from build123d import *

# Parameters (mm, degrees)
BOSS_EXTRUDE1_DEPTH            = 6.5
BOSS_EXTRUDE1_DEPTH_BACK       = 3.75
SKETCH1_W                      = 36
SKETCH1_H                      = 48
SKETCH2_W                      = 56
SKETCH2_H                      = 48
BOSS_EXTRUDE2_DEPTH            = 3.75
CBORE_FOR_M3_SHCS1_D           = 3.4
CBORE_FOR_M3_SHCS1_DEPTH       = 10.1
CBORE_FOR_M3_SHCS1_CBORE_D     = 6.5
CBORE_FOR_M3_SHCS1_CBORE_DEPTH = 3
CBORE_FOR_M3_SHCS1_TIP         = 1.021463052
CUT_EXTRUDE1_DEPTH             = 15.25
LPATTERN1_COUNT                = 2
LPATTERN1_PITCH                = 18


with BuildPart() as part:
    # Sketch1 → Boss-Extrude1 (new, two sides: drawn at the far end of the back side and taken through both)
    with BuildSketch(Plane.XY.offset(-BOSS_EXTRUDE1_DEPTH_BACK)):
        Rectangle(SKETCH1_W, SKETCH1_H)
    extrude(amount=BOSS_EXTRUDE1_DEPTH + BOSS_EXTRUDE1_DEPTH_BACK)

    # Sketch2 → Boss-Extrude2 (add)
    with BuildSketch(Plane(origin=(0, 0, 6.5), x_dir=(-1, 0, 0), z_dir=(0, 0, -1))):
        Rectangle(SKETCH2_W, SKETCH2_H)
    extrude(amount=BOSS_EXTRUDE2_DEPTH)

    # CBORE for M3 SHCS1
    with Locations(Plane.XY.offset(6.5)):
        with Locations((-23.5, 17), (-23.5, -17), (23.5, 17), (23.5, -17)):
            CounterBoreHole(CBORE_FOR_M3_SHCS1_D / 2, CBORE_FOR_M3_SHCS1_CBORE_D / 2, CBORE_FOR_M3_SHCS1_CBORE_DEPTH, depth=CBORE_FOR_M3_SHCS1_DEPTH)
            with Locations((0, 0, -(CBORE_FOR_M3_SHCS1_DEPTH + CBORE_FOR_M3_SHCS1_TIP / 2))):  # 118° drill point
                Cone(0, CBORE_FOR_M3_SHCS1_D / 2, CBORE_FOR_M3_SHCS1_TIP, mode=Mode.SUBTRACT)

    # Sketch7 → Cut-Extrude1 (cut)
    with BuildSketch(Plane(origin=(16.5, 0, 0), x_dir=(0, 0, -1), z_dir=(1, 0, 0))):
        Polygon((-6.503383917, 8.006767833), (-3.756779362, 8.006767833), (-3.756779362, 9.003383917), (2.246616083, 9.003383917), (2.246616083, 7.503383917), (3.746616083, 7.503383917), (6.355468839, 7.503383917), (6.355468839, -12.746616083), (3.871124209, -12.746616083), (3.746616083, -12.746616083), (2.246616083, -12.746616083), (2.246616083, -14.496616083), (-3.756779362, -14.496616083), (-3.756779362, -9.25), (-6.503383917, -9.25), align=None)
    cut_extrude1 = extrude(amount=-CUT_EXTRUDE1_DEPTH, mode=Mode.SUBTRACT)

    # LPattern1: Cut-Extrude1 ×2
    with Locations(*[(-i * LPATTERN1_PITCH, 0, 0) for i in range(1, LPATTERN1_COUNT)]):
        add(cut_extrude1, mode=Mode.SUBTRACT)


solid = part.part
Can you work these out from the model? Positions are in its coordinate system, mm. A direction names the side the tool comes from. Round coordinates to 2 decimals unless told otherwise and drop trailing zeros. Order: outer loops, then holes, each group sorted by start corner. A loop starts at its lowest first (then second) coordinate and runs counter-clockwise, first axis right, second up. Notation, with made-up numbers: M 59.5,32.5 L 93.5,32.5 A19 cw 93.5,64.5 Z; hole C -38.75,27.25 d7. An arc over 180 degrees is marked long. Use a Markdown table: item, result.
1) Imagine slicing it at A-A (y = -0.5). List the corners of the cut face in (x, z) for me, then the cut area to 3 significant figures.
Geometry says:
| item | result |
|---|---|
| outline | M -28,2.75 L -18,2.75 L -18,-3.75 L -16.75,-3.75 L -16.75,6.5 L -28,6.5 Z; M -1.5,-3.75 L 1.25,-3.75 L 1.25,6.5 L -1.5,6.5 Z; M 16.5,-3.75 L 18,-3.75 L 18,2.75 L 28,2.75 L 28,6.5 L 16.5,6.5 Z |
| area | 131 mm² |
2) If we mould it in two halves opening along Y, with no side actions, what happens to faces 1 (the face through (-22.1, 15.6, 3.5)), 2 (the face through (28, 0, 5)), 3 (the face through (-9, 9.003, 1))? For each: +Y half, -Y half, draft (parallel to the pull), parting line (faces both ways), or undercut.
Geometry says:
| item | result |
|---|---|
| face 1 | undercut |
| face 2 | draft |
| face 3 | undercut |
3) Imagine slicing it at B-B (x = -23.5). List the corners of the cut face in (y, z) for me.
Geometry says:
| item | result |
|---|---|
| outline | M -24,2.75 L -18.7,2.75 L -18.7,3.5 L -20.25,3.5 L -20.25,6.5 L -24,6.5 Z; M -15.3,2.75 L 15.3,2.75 L 15.3,3.5 L 13.75,3.5 L 13.75,6.5 L -13.75,6.5 L -13.75,3.5 L -15.3,3.5 Z; M 18.7,2.75 L 24,2.75 L 24,6.5 L 20.25,6.5 L 20.25,3.5 L 18.7,3.5 Z |
4) If I drill on line 1 along X through (y, z) = (5.5, -0.25); line 2 along Y through (x, z) = (23.5, 3.25); line 3 along Y through (x, z) = (-12, 1.75), over which ranges is the centre line in solid material (lowest first)?
Geometry says:
| item | result |
|---|---|
| line 1 | x = -18 to -16.75, -1.5 to 1.25, 16.5 to 18 |
| line 2 | y = -24 to -18.7, -15.3 to 15.3, 18.7 to 24 |
| line 3 | y = -24 to -14.5, 9 to 24 |
5) On a 3-axis mill with a long thin cutter (end or side, diameter ignored), from which of +Z, -Z, +X, -X, +Y, -Y can I reach the whole of each face in a straight line? I mean faces 4 (the face through (18, 0, -1)), 5 (the face through (-9, 8.007, 5)), 6 (the face through (9, -12.747, -3)), 7 (the face through (-9, -9.25, 5)), 8 (the face through (9, 8, -2.247)). Say none if no direction works.
Geometry says:
| item | result |
|---|---|
| face 4 | -Z, +X, +Y, -Y |
| face 5 | +Z |
| face 6 | -Z |
| face 7 | +Z, -Z |
| face 8 | none |
6) Imagine slicing it at D-D (z = 5.25). List the corners of the cut face in (x, y) for me, then the cut area to 3 significant figures.
Geometry says:
| item | result |
|---|---|
| outline | M -28,-24 L 28,-24 L 28,24 L -28,24 Z; hole C -23.5,-17 d6.5; hole C -23.5,17 d6.5; hole M -16.75,-9.25 L -1.5,-9.25 L -1.5,8.01 L -16.75,8.01 Z; hole M 1.25,-9.25 L 16.5,-9.25 L 16.5,8.01 L 1.25,8.01 Z; hole C 23.5,-17 d6.5; hole C 23.5,17 d6.5 |
| area | 2,030 mm² |
7) Imagine slicing it at C-C (x = -7.5). List the corners of the cut face in (y, z) for me, then the cut area to 3 significant figures.
Geometry says:
| item | result |
|---|---|
| outline | M -24,-3.75 L -12.75,-3.75 L -12.75,-2.25 L -14.5,-2.25 L -14.5,3.76 L -9.25,3.76 L -9.25,6.5 L -24,6.5 Z; M 7.5,-3.75 L 24,-3.75 L 24,6.5 L 8.01,6.5 L 8.01,3.76 L 9,3.76 L 9,-2.25 L 7.5,-2.25 Z |
| area | 273 mm² |
8) I'm going to push flat-ended pins straight in: P1, Ø3, axis at y = -12.5, z = 0, coming from the +X side; P2, Ø4, axis at x = -23.5, y = 17, coming from the +Z side; P3, Ø1.5, axis at y = -3.5, z = -2.5, coming from the -X side. Where does each tip first touch, or does it pass through?
Geometry says:
| item | result |
|---|---|
| P1 | stops at x = 18 |
| P2 | stops at z = 3.5 |
| P3 | stops at x = -18 |
